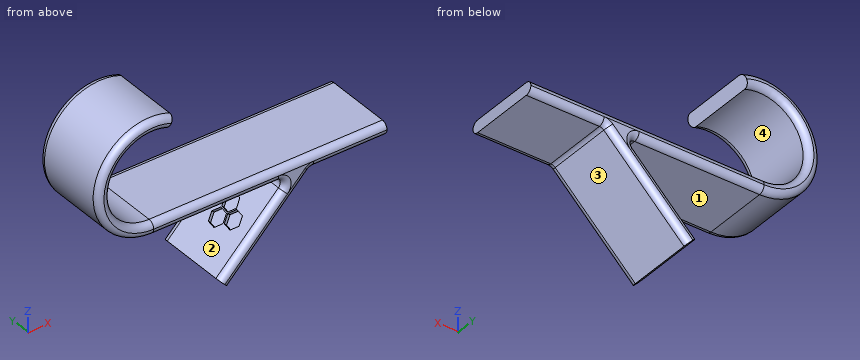
Autodesk Inventor part; units mm, degrees
ref_plane "YZ Plane" through (0, 0, 0) normal (1, 0, 0) x (0, 1, 0)
ref_plane "XZ Plane" through (0, 0, 0) normal (0, 1, 0) x (-1, 0, 0)
ref_plane "XY Plane" through (0, 0, 0) normal (0, 0, 1) x (1, 0, 0)
sketch "Sketch1" plane through (0, 0, 0) normal (0, 1, 0) x (-1, 0, 0)
  line L0 (0, -14) -> (-75, -14)
  line L1 (-75, -14) -> (-75, -18)
  line L2 (-4.7594, 13.1662) -> (-6.5571, 16.7632)
  arc A0 (0, -14) -> (-4.7594, 13.1662) centre (0, 0) ccw
  arc A1 (0, -18) -> (-6.5571, 16.7632) centre (0, 0) ccw
  line L3 (-45, -18) -> (-21.4678, -41.5322)
  line L4 (-45, -18) -> (-11.7204, -18) construction
  line L5 (-21.4678, -41.5322) -> (-24.2962, -44.3606)
  line L6 (-24.2962, -44.3606) -> (-50.6569, -18)
  line L7 (0, -18) -> (-45, -18)
  line L8 (-50.6569, -18) -> (-75, -18)
  point P0 (0, 0)
  dimension "d3" = 75
  dimension "d4" = 14
  dimension "d5" = 18
  dimension "d6" = 45
  dimension "d7" = 4
  dimension "d8" = 4
extrude "Extrusion1" add sketch "Sketch1" along normal blind 25
fillet "Fillet1" radius 2 12 edges at (-17.6881, 0, 3.3364) (22.5, 0, -18) (62.8284, 0, -18) (62.8284, 25, -18) (50.6569, 12.5, -18) (33.2339, 0, -29.7661) (37.4765, 0, -31.1803) (37.4765, 25, -31.1803) (33.2339, 25, -29.7661) (45, 12.5, -18) (-17.6881, 25, 3.3364) (22.5, 25, -18)
fillet "Fillet2" radius 2 4 edges at (37.5, 0, -14) (-13.79, 0, 2.4159) (-13.79, 25, 2.4159) (37.5, 25, -14)
sketch "Sketch2" plane through (0, 23, -14) normal (0, 0, 1) x (1, 0, 0)
  point P0 (0, -23)
sketch "Sketch3" plane through (0, 23, -14) normal (0, 0, 1) x (1, 0, 0)
  point P0 (0, -23)
sketch "Sketch4" plane through (41.5858, 2, -21.4142) normal (-0.7071, 0, 0.7071) x (0.7071, 0, 0.7071)
  line L0 (-28.4512, 21) -> (0, 21)
  line L1 (-17.898, 13.2543) -> (-15.2412, 14.305)
  line L2 (-15.2412, 14.305) -> (-13.0028, 12.5295)
  line L3 (-13.0028, 12.5295) -> (-13.4212, 9.7033)
  line L4 (-13.4212, 9.7033) -> (-16.078, 8.6525)
  line L5 (-16.078, 8.6525) -> (-18.3165, 10.428)
  line L6 (-18.3165, 10.428) -> (-17.898, 13.2543)
  line L7 (-12.6348, 12.4651) -> (-9.978, 13.5159)
  line L8 (-9.978, 13.5159) -> (-7.7396, 11.7404)
  line L9 (-7.7396, 11.7404) -> (-8.158, 8.9141)
  line L10 (-8.158, 8.9141) -> (-10.8148, 7.8633)
  line L11 (-10.8148, 7.8633) -> (-13.0532, 9.6388)
  line L12 (-13.0532, 9.6388) -> (-12.6348, 12.4651)
  line L13 (-15.916, 8.2429) -> (-13.2592, 9.2936)
  line L14 (-13.2592, 9.2936) -> (-11.0208, 7.5181)
  line L15 (-11.0208, 7.5181) -> (-11.4392, 4.6919)
  line L16 (-11.4392, 4.6919) -> (-14.096, 3.6411)
  line L17 (-14.096, 3.6411) -> (-16.3345, 5.4166)
  line L18 (-16.3345, 5.4166) -> (-15.916, 8.2429)
  point P0 (-14.2635, -2)
  point P1 (-12.0615, 16.231)
extrude "Extrusion2" cut sketch "Sketch4" against normal blind 1 and the other way blind 5
properties part number "TubeRadiator"
The model under review builds one solid part; all positions refer to its coordinate system, in mm. Face numbers are marked on the shaded views. Round coordinates to 2 decimals unless told otherwise and drop trailing zeros. Order: outer loops, then holes, each group sorted by start corner. A loop starts at its lowest first (then second) coordinate and runs counter-clockwise, first axis right, second up. Notation, with made-up numbers: (27.25, 77.5) -> (67.25, 77.5) arc R21 cw to (67.25, 100.5) -> close; hole circle Ø1 at (-7.5, 87). An arc over 180 degrees is marked (long way). Return JSON: item names as keys, results as strings.
1. Take a section at A-A (y = 21). Write out the cut boundary in (x, z), then the cut area to 3 significant figures.
Answer block:
{"outline": "(0, -18) -> (40.17, -18) arc R2 cw to (41.59, -21.41) -> (21.47, -41.53) -> (24.3, -44.36) -> (50.07, -18.59) arc R2 cw to (51.49, -18) -> (75, -18) -> (75, -14) -> (0, -14) arc R14 cw (long way) to (4.76, 13.17) -> (6.56, 16.76) arc R18 ccw (long way) to start", "area": "670 mm²"}
2. For L1, parallel to Z at x = 52.5, y = 14; L2, parallel to Z at x = -5, y = 4; L3, parallel to X at y = 22.25, z = -28.5, list the stretches that pass through material, from the lowest coordinate up. Write a range as [from, to].
Answer block:
{"L1": "z = [-18, -14]", "L2": "z = [-17.29, -13.08], [13.08, 17.29]", "L3": "x = [34.5, 40.16]"}
3. Insertion check: P1, Ø1.5, axis at x = 49.5, z = -19.5, coming from the +Y side; P2, Ø2, axis at x = 9.5, y = 18.5, coming from the +Z side; P3, Ø1, axis at x = 19, z = -19, coming from the -Y side; P4, Ø4, axis at x = 29.5, z = -13, coming from the -Y side. Each pin has a flat end and moves straight along its axis. Give the tip position at first contact, or say it passes through.
Answer block:
{"P1": "stops at y = 24.33", "P2": "stops at z = -14", "P3": "passes through", "P4": "stops at y = 0.27"}
4. The part is to be moulded in two halves that separate along X. For the marked faces 1, 2, 3 and 4, say which applies: +X half, -X half, draft (parallel to the pull), parting line (faces both ways), or undercut.
Answer block:
{"face 1": "draft", "face 2": "-X half", "face 3": "+X half", "face 4": "undercut"}
